```python
from build123d import *

# Parameters (mm, degrees)
SKETCH_1_W                  = 100
SKETCH_1_H                  = 75
EXTRUDE_1_DEPTH             = 1
SKETCH_2_R                  = 1.6
CUT_EXTRUDE_1_DEPTH         = 1
PATTERN_LINEAR_1_COUNT      = 2
PATTERN_LINEAR_1_PITCH      = 75
PATTERN_LINEAR_1_COUNT_DIR2 = 2
PATTERN_LINEAR_1_PITCH_DIR2 = 62


with BuildPart() as part:
    # ｽｹｯﾁ1 → ﾎﾞｽ - 押し出し1 (new body)
    with BuildSketch(Plane.XY):
        Rectangle(SKETCH_1_W, SKETCH_1_H)
    extrude(amount=EXTRUDE_1_DEPTH)

    # ｽｹｯﾁ2 → ｶｯﾄ - 押し出し1 (cut)
    with BuildSketch(Plane.XY.offset(1)):
        with Locations((42, -30.5)):
            Circle(SKETCH_2_R)
    cut_extrude_1 = extrude(amount=-CUT_EXTRUDE_1_DEPTH, mode=Mode.SUBTRACT)

    # 直線ﾊﾟﾀｰﾝ1: Cut-Extrude 1 2 × 2
    with Locations(*[(-i * PATTERN_LINEAR_1_PITCH, j * PATTERN_LINEAR_1_PITCH_DIR2, 0) for i in range(PATTERN_LINEAR_1_COUNT) for j in range(PATTERN_LINEAR_1_COUNT_DIR2) if (i, j) != (0, 0)]):
        add(cut_extrude_1, mode=Mode.SUBTRACT)


solid = part.part
```
Input: part model. Units: mm. Frame: model coordinates. Give positions to 0.01 mm unless a question says otherwise; leave off trailing zeros. Order: outer loops, then holes, each group sorted by start corner. A loop starts at its lowest first (then second) coordinate and runs counter-clockwise, first axis right, second up. Notation, with made-up numbers: (89.5, -32) -> (97.5, -32) arc R16 cw to (97.5, -20) -> close; hole circle Ø5 at (82, 89.5). An arc over 180 degrees is marked (long way). Write each question's results on one line, items separated by ' | '. Start each with the question number.
Item 1: Contact query for a flat-ended pin moving along its axis: P1, Ø5, axis at x = -33, y = -30.5, coming from the +Z side. Output: stop coordinate, or through.
Item 2: Cut plane A-A on y = 31.5. Return the cut outline in (x, z), then the cut area to 3 significant figures.
Item 3: Mould query, pull axis Y, two halves, no side actions, for faces 1 (the cylindrical face through (-34.27, 30.53, 0.51)), 2 (the flat face through (-1, 1, 0)). Classes: pulls with the +Y half, pulls with the -Y half, needs draft (parallel to the pull), parting line crosses it, or undercut.
Item 4: Line query: line 1 (Y direction, x = -33, z = 0.45). Output: solid intervals per line, ascending.
Item 5: Cut plane B-B on x = -33. Return the cut outline in (y, z), then the cut area to 3 significant figures.
Established:
1) P1: z = 1
2) outline: (-50, 0) -> (-34.6, 0) -> (-34.6, 1) -> (-50, 1) -> close; (-31.4, 0) -> (40.4, 0) -> (40.4, 1) -> (-31.4, 1) -> close; (43.6, 0) -> (50, 0) -> (50, 1) -> (43.6, 1) -> close | area: 93.6 mm^2
3) face 1: undercut | face 2: needs draft
4) line 1: -37.5 to -32.1, -28.9 to 29.9, 33.1 to 37.5
5) outline: (-37.5, 0) -> (-32.1, 0) -> (-32.1, 1) -> (-37.5, 1) -> close; (-28.9, 0) -> (29.9, 0) -> (29.9, 1) -> (-28.9, 1) -> close; (33.1, 0) -> (37.5, 0) -> (37.5, 1) -> (33.1, 1) -> close | area: 68.6 mm^2
